from build123d import *
from build123d.topology import SkipClean

# Parameters (mm, degrees)
SKETCH_1_R          = 6
EXTRUDE_1_DEPTH     = 150
SKETCH_2_R          = 8
EXTRUDE_2_DEPTH     = 5
EXTRUDE_START       = 30
SKETCH_3_R          = 6
EXTRUDE_5_DEPTH     = 30
SKETCH_9_W          = 19.221444034
SKETCH_9_H          = 5.745349359
CUT_EXTRUDE_7_DEPTH = 40
FILLET_4_R          = 5
FILLET_5_R          = 5


with BuildPart() as part:
    # 草图1 → 凸台-拉伸1 (new body)
    with BuildSketch(Plane.XY):
        Circle(SKETCH_1_R)
    extrude(amount=EXTRUDE_1_DEPTH)

    # 草图2 → 凸台-拉伸2 (add)
    with BuildSketch(Plane.XY):
        Circle(SKETCH_2_R)
    extrude(amount=-EXTRUDE_2_DEPTH)

    # 草图3 → 凸台-拉伸5 (add)
    with BuildSketch(Plane(origin=(0, 0, -5), x_dir=(-1, 0, 0), z_dir=(0, 0, -1)).offset(EXTRUDE_START)):
        with Locations(Location((0, 0, 0), (0, 0, 180))):
            Circle(SKETCH_3_R)
    extrude(amount=-EXTRUDE_5_DEPTH)

    # 草图8 one side → 旋转8 (revolve)
    with SkipClean():  # the faces are left unmerged after this step: merging them gives an invalid solid
        with BuildSketch(Plane(origin=(0, 0, -35), x_dir=(-1, 0, 0), z_dir=(0, 0, -1))):
            with BuildLine():
                Line((0, 6), (0, -6))
                ThreePointArc((0, -6), (4.242640687, -4.242640687), (6, 0))
                ThreePointArc((6, 0), (4.242640687, 4.242640687), (0, 6))
            make_face()
        revolve(axis=Axis((0, 0, -35), (0, -1, 0)))

    # 草图9 → 切除-拉伸7 (cut)
    with BuildSketch(Plane(origin=(0, 0, -9), x_dir=(-1, 0, 0), z_dir=(0, 0, -1))):
        with Locations((0.738599267, 4.336128304)):
            Rectangle(SKETCH_9_W, SKETCH_9_H)
        with Locations((0.738599267, -4.336128304)):
            Rectangle(SKETCH_9_W, SKETCH_9_H)
    extrude(amount=CUT_EXTRUDE_7_DEPTH, mode=Mode.SUBTRACT)

    # 圆角4
    # the kernel refuses this fillet: 5 mm, written as the material it adds along each edge
    with BuildSketch(Plane(origin=(18.318788834, 1.463453624, -9), x_dir=(0, 0, -1), z_dir=(-1, 0, 0))) as fillet_4_piece_1_section:
        with BuildLine():
            CenterArc((FILLET_4_R, -FILLET_4_R), FILLET_4_R, 90, 90)
            Line((0, -FILLET_4_R), (0, 0))
            Line((0, 0), (FILLET_4_R, 0))
        make_face()
    fillet_4_piece_1 = extrude(amount=36.637577667, mode=Mode.PRIVATE)
    fillet_4_piece_1 = fillet_4_piece_1 & Plane(origin=(0, 0, -10.216169301), x_dir=(1, 0, 0), z_dir=(0, 0, -1)) * Cylinder(6, 94, mode=Mode.PRIVATE)
    add(fillet_4_piece_1)

    # 圆角5
    # the kernel refuses this fillet: 5 mm, written as the material it adds along each edge
    with BuildSketch(Plane(origin=(18.318788834, -1.463453624, -9), x_dir=(0, 0, -1), z_dir=(-1, 0, 0))) as fillet_5_piece_1_section:
        with BuildLine():
            CenterArc((FILLET_5_R, FILLET_5_R), FILLET_5_R, 180, 90)
            Line((0, FILLET_5_R), (0, 0))
            Line((0, 0), (FILLET_5_R, 0))
        make_face()
    fillet_5_piece_1 = extrude(amount=36.637577667, mode=Mode.PRIVATE)
    fillet_5_piece_1 = fillet_5_piece_1 & Plane(origin=(0, 0, -10.216169301), x_dir=(1, 0, 0), z_dir=(0, 0, -1)) * Cylinder(6, 94, mode=Mode.PRIVATE)
    add(fillet_5_piece_1)


solid = part.part
Model file for the job. Use its own axes, mm. A direction names the side the tool comes from. Coordinates: 2 decimals unless noted, no trailing zeros. Write each loop counter-clockwise with the first axis right and the second up, starting at its lowest first coordinate (ties: lowest second). Pieces come first, ordered by that corner, then holes. Notation, with made-up numbers: (0, -20.75) -> (5, -20.75) arc R11 cw to (5, -8.75) -> close; hole circle Ø9 at (45, 37.5). An arc over 180 degrees is marked (long way). One line per item, written item: value. Start each with the question number.
1) Slice it at B-B on z = 76. Write the cut outline in (x, y).
2) Which spindle directions (+Z, -Z, +X, -X, +Y, -Y) get a long thin tool onto all of the face, cutting with end or side? Do faces 1 (the face through (-2, 6, 0)), 2 (the face through (-2, 6, -5)), 3 (the face through (0, -1.463, -27)). Say none if no direction does.
3) Probe probe 1 along Y at (x, z) = (0.5, 126); probe 2 along Z at (x, y) = (4.5, -5); probe 3 along Y at (x, z) = (-1.5, -23). List the from-to ranges inside material, lowest first.
4) Slice it at A-A on x = 0. Write the cut outline in (y, z), then the cut area to 3 significant figures.
5) Flat gauge pins, fed straight in: pin 1 Ø1 at (y, z) = (3, 16) entering from -X; pin 2 Ø8 at (x, y) = (1, 3) entering from -Z; pin 3 Ø9.5 at (x, z) = (2, -22.5) entering from +Y; pin 4 Ø3 at (x, y) = (-2.5, 1.5) entering from -Z. Where does each tip first touch, or does it go through?
Answers follow:
1. outline: circle Ø12 at (0, 0)
2. face 1: +Z
2. face 2: -Z
2. face 3: -Z, +X, -X, -Y
3. probe 1: -5.98 to 5.98
3. probe 2: -5 to 0
3. probe 3: -1.46 to 1.46
4. outline: (-8, -5) -> (-6, -5) -> (-6, -9.02) arc R5 cw to (-1.46, -14) -> (-1.46, -40.82) arc R6 ccw to (1.46, -40.82) -> (1.46, -14) arc R5 cw to (6, -9.02) -> (6, -5) -> (8, -5) -> (8, 0) -> (6, 0) -> (6, 150) -> (-6, 150) -> (-6, 0) -> (-8, 0) -> close
4. area: 2,030 mm2
5. pin 1: x = -5.45
5. pin 2: z = -41
5. pin 3: y = 1.46
5. pin 4: z = -40.83
